Geometry: final body of the model. Coordinates: model frame, mm. A direction names the side the tool comes from. Round coordinates to 2 decimals unless told otherwise and drop trailing zeros. Loops run counter-clockwise (first coordinate to the right, second up) from the corner with the lowest first, then second, coordinate; pieces in that order, holes last. Notation, with made-up numbers: M 46,14 L 97,14 A22 ccw 97,36 Z; hole C -29.5,1 d4. An arc over 180 degrees is marked long. Write each question's results on one line, items separated by ' | '.
```python
from build123d import *

# Parameters (mm, degrees)
SKETCH1_R             = 30
BOSS_EXTRUDE1_DEPTH   = 30
F_6_0MM_DOWEL_HOLE1_D = 6
SKETCH2_R             = 11
BOSS_EXTRUDE2_DEPTH   = 10
SKETCH9_R             = 3.95
BOSS_EXTRUDE3_DEPTH   = 30
SKETCH10_R            = 10.25
CUT_EXTRUDE2_DEPTH    = 20.5
SKETCH12_R            = 3.2
CUT_EXTRUDE3_DEPTH    = 70


with BuildPart() as part:
    # Sketch1 → Boss-Extrude1 (new body)
    with BuildSketch(Plane.XY):
        Circle(SKETCH1_R)
    extrude(amount=BOSS_EXTRUDE1_DEPTH)

    # Ø6.0mm Dowel Hole1 (through all)
    with Locations(Plane.XY.offset(30)):
        with Locations((-15.733125881, 15.733125881), (15.733125881, -15.733125881), (-15.733125881, -15.733125881)):
            Hole(F_6_0MM_DOWEL_HOLE1_D / 2)

    # Sketch2 → Boss-Extrude2 (add)
    with BuildSketch(Plane.XY.offset(30)):
        Circle(SKETCH2_R)
    extrude(amount=BOSS_EXTRUDE2_DEPTH)

    # Sketch9 → Boss-Extrude3 (add)
    with BuildSketch(Plane.XY.offset(40)):
        with Locations((0, -3)):
            Circle(SKETCH9_R)
    extrude(amount=BOSS_EXTRUDE3_DEPTH)

    # Sketch10 → Cut-Extrude2 (cut)
    with BuildSketch(Plane(origin=(0, 0, 0), x_dir=(-1, 0, 0), z_dir=(0, 0, -1))):
        Circle(SKETCH10_R)
    extrude(amount=-CUT_EXTRUDE2_DEPTH, mode=Mode.SUBTRACT)

    # Sketch12 → Cut-Extrude3 (cut)
    with BuildSketch(Plane(origin=(0, 30, 0), x_dir=(1, 0, 0), z_dir=(0, 1, 0))):
        with Locations(Location((0, -11.5, 0), (0, 0, 270))):
            Circle(SKETCH12_R)
    extrude(amount=-CUT_EXTRUDE3_DEPTH, mode=Mode.SUBTRACT)


solid = part.part
```
1. Section A-A (x = 0). Output: boundary loops of the cut face in (y, z).
Answer key:
outline: M -30,0 L -10.25,0 L -10.25,8.3 L -30,8.3 Z; M -30,14.7 L -10.25,14.7 L -10.25,20.5 L 10.25,20.5 L 10.25,14.7 L 30,14.7 L 30,30 L 11,30 L 11,40 L 0.95,40 L 0.95,70 L -6.95,70 L -6.95,40 L -11,40 L -11,30 L -30,30 Z; M 10.25,0 L 30,0 L 30,8.3 L 10.25,8.3 Z
2. Section B-B (y = 23). Output: boundary loops of the cut face in (x, z).
Answer key:
outline: M -19.26,0 L 19.26,0 L 19.26,30 L -19.26,30 Z; hole C 0,11.5 d6.4
3. Draft query along Y for faces 4 (the face through (-1.226, -19.719, 14.456)), 5 (the face through (-15.1, 12.8, 14.8)), 6 (the face through (-2.91, -0.33, 54.79)), 7 (the face through (18.114, -17.559, 14.79)). Return one class per face: pulls with the +Y half, pulls with the -Y half, needs draft (parallel to the pull), parting line crosses it, or undercut.
Answer key:
face 4: needs draft | face 5: undercut | face 6: parting line crosses it | face 7: undercut
4. Section C-C (y = -6). Output: boundary loops of the cut face in (x, z).
Answer key:
outline: M -29.39,0 L -8.31,0 L -8.31,20.5 L 8.31,20.5 L 8.31,0 L 29.39,0 L 29.39,30 L 9.22,30 L 9.22,40 L 2.57,40 L 2.57,70 L -2.57,70 L -2.57,40 L -9.22,40 L -9.22,30 L -29.39,30 Z
5. Ray query, probe 1 along Z at (x, y) = (0, -20); probe 2 along Y at (x, z) = (-15.5, 28); probe 3 along Z at (x, y) = (-21.5, 8.5). Return the intervals inside material, ascending.
Answer key:
probe 1: z = 0 to 8.3, 14.7 to 30 | probe 2: y = -25.69 to -18.72, -12.74 to 12.74, 18.72 to 25.69 | probe 3: z = 0 to 30
6. Access query for faces 1 (the face through (-2.38, -10.74, 34.93)), 2 (the face through (-9.777, 3.079, 10.106)), 3 (the face through (0, -3, 70)). Directions: +Z, -Z, +X, -X, +Y, -Y. A direction counts if a zero-diameter tool reaches every point of the face in a straight line with its end or side. Return the directions, or none.
Answer key:
face 1: +Z | face 2: -Z | face 3: +Z, +X, -X, +Y, -Y
7. Pin query (flat end, axial travel): P1, Ø5.5, axis at x = -15.73, y = 15.73, coming from the -Z side; P2, Ø3, axis at x = 21, z = 24, coming from the -Y side; P3, Ø12, axis at x = -18.5, z = 21.5, coming from the -Y side; P4, Ø4, axis at x = -0.5, z = 57.5, coming from the +Y side. Return the tip coordinate at first contact, or that it passes through.
Answer key:
P1: passes through | P2: stops at y = -22.8 | P3: stops at y = -27.27 | P4: stops at y = 0.95
8. Section D-D (z = 57.5). Output: boundary loops of the cut face in (x, y), then the cut area to 3 significant figures.
Answer key:
outline: C 0,-3 d7.9 | area: 49.0 mm²
